```python
from build123d import *

# Parameters (mm, degrees)
F0_W     = 30
F0_H     = 25
F1_DEPTH = 20


with BuildPart() as f1:
    # F0 (on Right) → F1 (new body)
    with BuildSketch(Plane.YZ):
        Polygon((-62.467675, 54.630118), (-117.467675, 54.630118), (-117.467675, -60.369882), (-62.467675, -60.369882), (-67.467675, -40.369882), (-27.467675, -40.369882), (-32.467675, -60.369882), (22.532325, -60.369882), (17.532325, -40.369882), (57.532325, -40.369882), (52.532325, -60.369882), (107.532325, -60.369882), (102.532325, -40.369882), (142.532325, -40.369882), (137.532325, -60.369882), (192.532325, -60.369882), (192.532325, 54.630118), (137.532325, 54.630118), (107.532325, 54.630118), (52.532325, 54.630118), (22.532325, 54.630118), (-32.467675, 54.630118), align=None)
        with Locations((122.532325, 67.130118)):
            Rectangle(F0_W, F0_H)
        with Locations((37.532325, 67.130118)):
            Rectangle(F0_W, F0_H)
        with Locations((-47.467675, 67.130118)):
            Rectangle(F0_W, F0_H)
    extrude(amount=F1_DEPTH)


solid = f1.part
```
Input: part model. Units: mm. Frame: model coordinates. A direction names the side the tool comes from. Round coordinates to 2 decimals unless told otherwise and drop trailing zeros. Loops run counter-clockwise (first coordinate to the right, second up) from the corner with the lowest first, then second, coordinate; pieces in that order, holes last. Notation, with made-up numbers: M 68.25,53.5 L 101.25,53.5 A20 ccw 101.25,91.5 Z; hole C -34,63 d1. An arc over 180 degrees is marked long. Answer in a Markdown table with one row per item. Add a question column.
1. Section D-D (y = 82). Output: boundary loops of the cut face in (x, z), and give its area (3 significant figures).
2. Set-up query: faces 1 (the face through (10, 122, 79.63)), 2 (the face through (9.86, -29.933, -50.23)), 3 (the face through (10, -32.468, 67)), 4 (the face through (10, -90, 54.63)). Return all of +Z, -Z, +X, -X, +Y, -Y with unobstructed straight access to the full face (end or side cutting, diameter ignored); none if empty.
3. Mould query, pull axis Z, two halves, no side actions, for faces 5 (the face through (10, -90, -60.37)), 6 (the face through (10, 37, -40.37)), 7 (the face through (10, -5, 54.63)). Classes: released by +Z, released by -Z, zero draft, split by the parting line, or undercut.
4. Section B-B (x = 13.5). Output: boundary loops of the cut face in (y, z).
5. Section A-A (z = 59). Output: boundary loops of the cut face in (x, y).
6. Section C-C (z = -48). Output: boundary loops of the cut face in (x, y).
7. Ray query, probe 1 along Y at (x, z) = (9, 58); probe 2 along Y at (x, z) = (6.25, -49); probe 3 along Z at (x, y) = (5.5, 74.5). Return the intervals inside material, ascending.
8. Contact query for flat-ended pins moving along their axis: pin 1 (10 mm diameter, centred on x = 14, z = 71.5, fed in from +Y); pin 2 (6 mm diameter, centred on x = 11, y = -11.5, fed in from +Z); pin 3 (10 mm diameter, centred on x = 10.5, y = 37, fed in from -Z). Output: stop coordinate, or through.
Values follow:
| question | item | result |
|---|---|---|
| 1 | outline | M 0,-60.37 L 20,-60.37 L 20,54.63 L 0,54.63 Z |
| 1 | area | 2,300 mm^2 |
| 2 | face 1 | +Z, +X, -X, +Y, -Y |
| 2 | face 2 | +X, -X |
| 2 | face 3 | +Z, +X, -X |
| 2 | face 4 | +Z, +X, -X, -Y |
| 3 | face 5 | released by -Z |
| 3 | face 6 | undercut |
| 3 | face 7 | released by +Z |
| 4 | outline | M -117.47,-60.37 L -62.47,-60.37 L -67.47,-40.37 L -27.47,-40.37 L -32.47,-60.37 L 22.53,-60.37 L 17.53,-40.37 L 57.53,-40.37 L 52.53,-60.37 L 107.53,-60.37 L 102.53,-40.37 L 142.53,-40.37 L 137.53,-60.37 L 192.53,-60.37 L 192.53,54.63 L 137.53,54.63 L 137.53,79.63 L 107.53,79.63 L 107.53,54.63 L 52.53,54.63 L 52.53,79.63 L 22.53,79.63 L 22.53,54.63 L -32.47,54.63 L -32.47,79.63 L -62.47,79.63 L -62.47,54.63 L -117.47,54.63 Z |
| 5 | outline | M 0,-62.47 L 20,-62.47 L 20,-32.47 L 0,-32.47 Z; M 0,22.53 L 20,22.53 L 20,52.53 L 0,52.53 Z; M 0,107.53 L 20,107.53 L 20,137.53 L 0,137.53 Z |
| 6 | outline | M 0,-117.47 L 20,-117.47 L 20,-65.56 L 0,-65.56 Z; M 0,-29.38 L 20,-29.38 L 20,19.44 L 0,19.44 Z; M 0,55.62 L 20,55.62 L 20,104.44 L 0,104.44 Z; M 0,140.62 L 20,140.62 L 20,192.53 L 0,192.53 Z |
| 7 | probe 1 | -62.47 to -32.47, 22.53 to 52.53, 107.53 to 137.53 |
| 7 | probe 2 | -117.47 to -65.31, -29.63 to 19.69, 55.37 to 104.69, 140.37 to 192.53 |
| 7 | probe 3 | -60.37 to 54.63 |
| 8 | pin 1 | y = 137.53 |
| 8 | pin 2 | z = 54.63 |
| 8 | pin 3 | z = -40.37 |
